Autodesk Inventor part; units mm, degrees
ref_plane "YZ Plane" through (0, 0, 0) normal (1, 0, 0) x (0, 1, 0)
ref_plane "XZ Plane" through (0, 0, 0) normal (0, 1, 0) x (-1, 0, 0)
ref_plane "XY Plane" through (0, 0, 0) normal (0, 0, 1) x (1, 0, 0)
sketch "Sketch1" plane through (0, 0, 0) normal (0, 0, 1) x (1, 0, 0)
  circle A0 centre (0, 0) radius 1.1906
  dimension "d0" = 2.3813
extrude "Extrusion1" add sketch "Sketch1" along normal mid plane 9.525
chamfer "Chamfer1" distance 0.381 angle 45 2 edges at (-1.1906, 0, -4.7625) (-1.1906, 0, 4.7625)
scale "Scale1" factors (10, 10, 10) then translate (0, 0, 0) bodies 1
properties part number "hex axle pin"
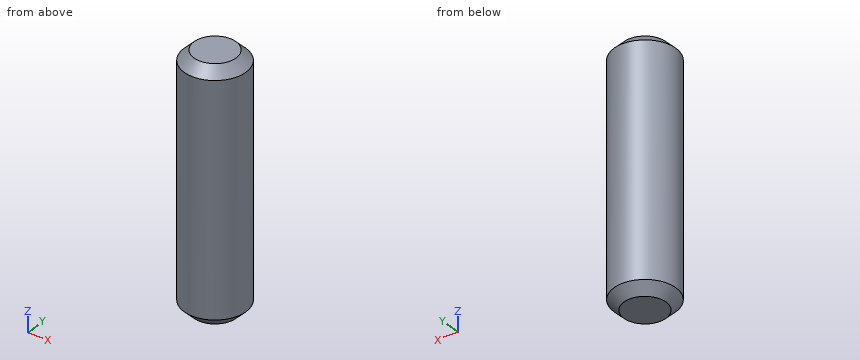
Build history of the part. All positions in model axes, mm. Round coordinates to 2 decimals unless told otherwise and drop trailing zeros. Loops run counter-clockwise (first coordinate to the right, second up) from the corner with the lowest first, then second, coordinate; pieces in that order, holes last.
Item 1: Saw through at A-A (z = 42.5). List the corners of the cut face in (x, y).
Item 2: Drill centre lines: line 1 along X through (y, z) = (-6, 1.5); line 2 along X through (y, z) = (8.25, 38.5); line 3 along Y through (x, z) = (-8, 2). Where is each one in solid material? Low to high.
Item 3: Pin check, flat tips, straight feed: P1, Ø2, axis at y = 7, z = -38, coming from the +X side; P2, Ø3, axis at x = -6, z = 28.5, coming from the +Y side; P3, Ø6, axis at y = -6, z = 27, coming from the -X side. Stop position of each tip, or through.
Worked answers:
1. outline: circle Ø23.81 at (0, 0)
2. line 1: x = -10.28 to 10.28
2. line 2: x = -8.58 to 8.58
2. line 3: y = -8.82 to 8.82
3. P1: stops at x = 10.28
3. P2: stops at y = 11.02
3. P3: stops at x = -11.52
